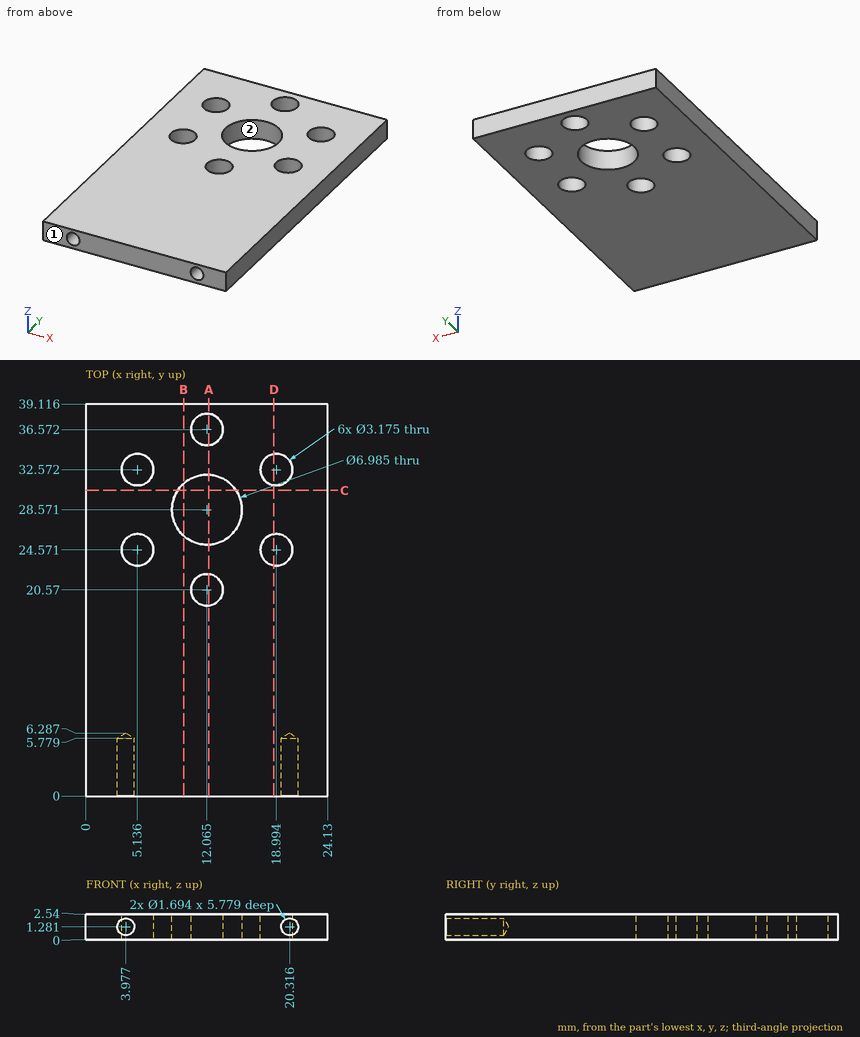
For this review, use the dimensioned drawing (mm, ordinates from the lowest corner) and the shaded views. Give positions to 0.01 mm unless a question says otherwise; leave off trailing zeros. Order: outer loops, then holes, each group sorted by start corner. A loop starts at its lowest first (then second) coordinate and runs counter-clockwise, first axis right, second up. Notation, with made-up numbers: (25.5, 68.5) - (43.5, 68.5) arc R22 cw to (43.5, 106.5) - close; hole circle Ø2 at (68.25, -5). An arc over 180 degrees is marked (long way). Use a Markdown table: item, result. Add a question column.
(1) Mouldability with a two-part tool opening along X and no side actions: class the marked faces 1 and 2 as +X half, -X half, draft (parallel to the pull), parting line (faces both ways), or undercut.
(2) Add section C-C on y = 30.5. Give the boundary of the cut face in (x, z).
(3) Wall thickness on probe 1 along Y at (x, z) = (12, 1.7) (1 decimal); probe 2 along Y at (x, z) = (4.25, 1.1) (1 decimal); probe 3 along X at (y, z) = (2.5, 1.65) (1 decimal): over which ranges is each line inside the solid? List them lowest first. Write a range as [from, to].
(4) Add section D-D on x = 18.75. Give the boundary of the cut face in (y, z) (1 decimal).
(5) Add section B-B on x = 9.75. Give the boundary of the cut face in (y, z) (1 decimal).
(6) Add section A-A on x = 12.25. Give the number of separate pieces and of enclosed holes in the cut face.
Report:
| question | item | result |
|---|---|---|
| 1 | face 1 | draft |
| 1 | face 2 | undercut |
| 2 | outline | (0, 0) - (9.15, 0) - (9.15, 2.54) - (0, 2.54) - close; (14.98, 0) - (24.13, 0) - (24.13, 2.54) - (14.98, 2.54) - close |
| 3 | probe 1 | y = [0, 19], [22.2, 25.1], [32.1, 35], [38.2, 39.1] |
| 3 | probe 2 | y = [6.1, 23.3], [25.9, 31.3], [33.9, 39.1] |
| 3 | probe 3 | x = [0, 3.2], [4.7, 19.6], [21.1, 24.1] |
| 4 | outline | (0, 0) - (23, 0) - (23, 2.5) - (0, 2.5) - close; (26.1, 0) - (31, 0) - (31, 2.5) - (26.1, 2.5) - close; (34.1, 0) - (39.1, 0) - (39.1, 2.5) - (34.1, 2.5) - close |
| 5 | outline | (0, 0) - (26, 0) - (26, 2.5) - (0, 2.5) - close; (31.2, 0) - (39.1, 0) - (39.1, 2.5) - (31.2, 2.5) - close |
| 6 | separate pieces | 4 |
| 6 | enclosed holes | 0 |
